Geometry: final body of the model. Coordinates: model frame, mm. Face numbers are marked on the shaded views. A direction names the side the tool comes from. Give positions to 0.01 mm unless a question says otherwise; leave off trailing zeros. Loops run counter-clockwise (first coordinate to the right, second up) from the corner with the lowest first, then second, coordinate; pieces in that order, holes last.
1. Draft query along Y for the marked faces 4, 5 and 6. Return one class per face: +Y half, -Y half, draft (parallel to the pull), parting line (faces both ways), or undercut.
2. Access query for the marked faces 1, 2 and 3. Directions: +Z, -Z, +X, -X, +Y, -Y. A direction counts if a zero-diameter tool reaches every point of the face in a straight line with its end or side. Return the directions, or none.
3. First-contact query: P1, Ø3, axis at x = 37, y = -5.72, coming from the -Z side; P2, Ø10.5, axis at y = -66.28, z = -10.17, coming from the +X side; P3, Ø10, axis at x = 21, y = -88, coming from the -Z side. Flat tips, straight axial feed; report the tip coordinate or a pass-through.
4. Material intervals for line 1 along Y through (x, z) = (37, 7.25); line 2 along Y through (x, z) = (20, -15); line 3 along Y through (x, z) = (38.5, -17.5), sorted ascending.
5. Section B-B, the plane z = -21.5. Output: boundary loops of the cut face in (x, y), then the cut area to 3 significant figures.
6. Section C-C, the plane y = -45. Output: boundary loops of the cut face in (x, z), then the cut area to 3 significant figures.
7. Section A-A, the plane x = 37. State how many separate pieces and enclosed holes the cut face has, then the cut area to 3 significant figures.
8. Section D-D, the plane x = 30.5. Output: boundary loops of the cut face in (y, z), then the cut area to 3 significant figures.
from build123d import *

# Parameters (mm, degrees)
F0_W         = 92
F0_H         = 48
F1_DEPTH     = 4
F2_R         = 3.25
F2_R_2       = 10.6786712851
F3_DEPTH     = 25
F4_W         = 9
F4_H         = 11
F4_H_2       = 3
F5_DEPTH     = 37.5
F6_R         = 2
F7_DEPTH     = 40
F8_W         = 0.1783174183
F8_H         = 5
F8_W_2       = 4.8216825817
F8_W_3       = 5
F9_DEPTH     = 3
F10_T4_DEPTH = 5
F12_DEPTH    = 9
F14_DEPTH    = 9


# Not quite as in the source:
# - a fillet or chamfer that OpenCascade refuses, or shapes differently, is made with other operations: its cross-section is extruded or revolved along the edge and cut away or added


with BuildPart() as f1:
    # F0 (on Right) → F1 (new body)
    with BuildSketch(Plane.YZ):
        with Locations((-47.0313817766, -16.1659868658)):
            Rectangle(F0_W, F0_H)
    extrude(amount=F1_DEPTH)

    # F2 (on face) → F3 (cut)
    with BuildSketch(Plane.YZ.offset(4)):
        with Locations((-66.2813817766, -10.1659868658)):
            Circle(F2_R)
        with Locations((-27.7813817766, -10.1659868658)):
            Circle(F2_R)
        with Locations((-66.2813817766, -33.2659868658)):
            Circle(F2_R)
        with Locations((-27.7813817766, -33.2659868658)):
            Circle(F2_R)
        with Locations((-47.217734158, -17.3795577139)):
            Circle(F2_R_2)
    extrude(amount=-F3_DEPTH, mode=Mode.SUBTRACT)

    # F4 (on face) → F5 (join)
    with BuildSketch(Plane.YZ.offset(4)):
        with Locations((-88.5313817766, -18.6659868658)):
            Rectangle(F4_W, F4_H)
        with Locations((-5.5313817766, -18.6659868658)):
            Rectangle(F4_W, F4_H)
        with Locations((-88.5313817766, 6.3340131342)):
            Rectangle(F4_W, F4_H_2)
        with Locations((-5.5313817766, 6.3340131342)):
            Rectangle(F4_W, F4_H_2)
    extrude(amount=F5_DEPTH)

    # F6 (on face) → F7 (cut)
    with BuildSketch(Plane.XY.offset(7.8340131342)):
        with Locations((37, -5.7174442336)):
            Circle(F6_R)
        with Locations((37, -87.7174442336)):
            Circle(F6_R)
    extrude(amount=-F7_DEPTH, mode=Mode.SUBTRACT)

    # F8 (on face) → F9 (cut)
    with BuildSketch(Plane(origin=(0, 0, 0), x_dir=(0, -1, 0), z_dir=(-1, 0, 0))):
        with Locations((0.9422230674, -21.7159868658)):
            Rectangle(F8_W, F8_H)
        with Locations((3.4422230674, -21.7159868658)):
            Rectangle(F8_W_2, F8_H)
        with Locations((90.5313817766, -21.7159868658)):
            Rectangle(F8_W_3, F8_H)
    extrude(amount=-F9_DEPTH, mode=Mode.SUBTRACT)

    # F10: chamfer of 5 on 1 edges, made by hand


with BuildPart() as f10_tool2:
    # F10_s3 → F10_t4 (new body)
    with BuildSketch(Plane.XY.offset(-19.2159868658)):
        Polygon((8, -1.0313817766), (3, -6.0313817766), (3, -1.0313817766), align=None)
    extrude(amount=-F10_T4_DEPTH)

    split(bisect_by=Plane.XZ.offset(5.8530643582), keep=Keep.BOTTOM)


with BuildPart() as f1_1:
    add(f1.part)

    # F10_t1: cut F10_tool2
    add(f10_tool2.part, mode=Mode.SUBTRACT)

    # F11 (on face) → F12 (join)
    with BuildSketch(Plane(origin=(0, -1.0313817766, 0), x_dir=(-1, 0, 0), z_dir=(0, 1, 0))):
        with BuildLine():
            ThreePointArc((-8, 4.8340131342), (-5.539111548, 3.2949015862), (-4, 0.8340131342))
            Line((-4, 0.8340131342), (-4, 4.8340131342))
            Line((-4, 4.8340131342), (-8, 4.8340131342))
        make_face()
    extrude(amount=-F12_DEPTH)

    # F13 (on face) → F14 (join)
    with BuildSketch(Plane.XZ.offset(93.0313817766)):
        with BuildLine():
            ThreePointArc((4, 0.8340131342), (5.7533122895, 3.408733727), (8.5231261328, 4.8340131342))
            Line((8.5231261328, 4.8340131342), (4, 4.8340131342))
            Line((4, 4.8340131342), (4, 0.8340131342))
        make_face()
    extrude(amount=-F14_DEPTH)


solid = f1_1.part
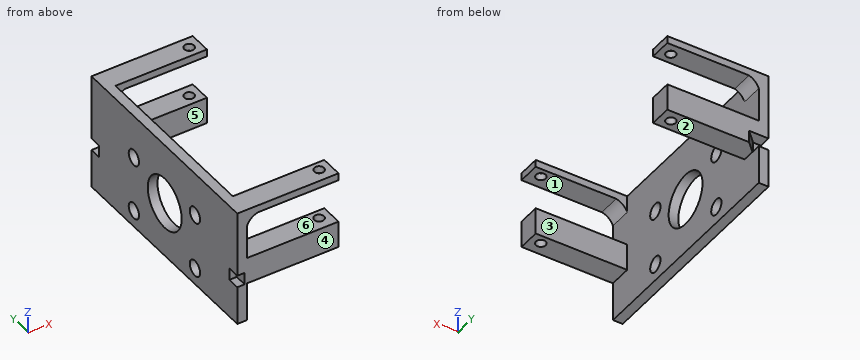
Answers below:
1. face 4: -Y half
1. face 5: undercut
1. face 6: draft
2. face 1: +X, +Y, -Y
2. face 2: -Z, +X, +Y, -Y
2. face 3: +Z, -Z, +X
3. P1: passes through
3. P2: stops at x = 4
3. P3: stops at z = -24.17
4. line 1: y = -93.03 to -89.72, -85.72 to -84.03, -10.03 to -7.72, -3.72 to -1.03
4. line 2: y = -93.03 to -84.03, -10.03 to -1.03
4. line 3: y = -93.03 to -89.04, -86.39 to -84.03, -10.03 to -7.04, -4.39 to -1.03
5. outline: (0, -88.03) - (3, -88.03) - (3, -93.03) - (41.5, -93.03) - (41.5, -84.03) - (4, -84.03) - (4, -57.07) - (0, -57.07) - close; (0, -37.37) - (4, -37.37) - (4, -10.03) - (41.5, -10.03) - (41.5, -1.03) - (8, -1.03) - (3.18, -5.85) - (0, -5.85) - close; hole circle Ø4 at (37, -87.72); hole circle Ø4 at (37, -5.72)
5. area: 897 mm2
6. outline: (0, -40.17) - (4, -40.17) - (4, -27.83) - (0, -27.83) - close; (0, -6.93) - (4, -6.93) - (4, 7.83) - (0, 7.83) - close
6. area: 108 mm2
7. separate pieces: 8
7. enclosed holes: 0
7. area: 140 mm2
8. outline: (-93.03, -24.17) - (-84.03, -24.17) - (-84.03, -13.17) - (-93.03, -13.17) - close; (-93.03, 4.83) - (-84.03, 4.83) - (-84.03, 7.83) - (-93.03, 7.83) - close; (-10.03, -24.17) - (-1.03, -24.17) - (-1.03, -13.17) - (-10.03, -13.17) - close; (-10.03, 4.83) - (-1.03, 4.83) - (-1.03, 7.83) - (-10.03, 7.83) - close
8. area: 252 mm2
